Can you work these out from the model? Positions are in its coordinate system, mm. A direction names the side the tool comes from. Give positions to 0.01 mm unless a question says otherwise; leave off trailing zeros. Write each loop counter-clockwise with the first axis right and the second up, starting at its lowest first coordinate (ties: lowest second). Pieces come first, ordered by that corner, then holes. Notation, with made-up numbers: (32, 22.25) -> (44, 22.25) arc R15 ccw to (44, 35.25) -> close; hole circle Ø10 at (83.5, 72.5). An arc over 180 degrees is marked (long way). One line per item, written item: value.
from build123d import *

# Parameters (mm, degrees)
BOSS_EXTRUDE1_DEPTH     = 35
BOSS_EXTRUDE2_START     = 3
BOSS_EXTRUDE2_DEPTH     = 3
CUT_EXTRUDE1_DEPTH      = 54.037722425
CUT_EXTRUDE1_DEPTH_BACK = 54.037722425
CUT_EXTRUDE2_START      = -3
CUT_EXTRUDE2_DEPTH      = 6
CHAMFER1_SIZE           = 1


with BuildPart() as part:
    # Sketch1 → Boss-Extrude1 (new body)
    with BuildSketch(Plane(origin=(0, 0, 0), x_dir=(1, 0, 0), z_dir=(0, 1, 0))):
        with BuildLine():
            Line((7, 25.5), (7, 35.5))
            ThreePointArc((7, 35.5), (9.5, 38), (12, 35.5))
            Line((12, 35.5), (12, 10.5))
            ThreePointArc((12, 10.5), (11.827182716, 8.470776255), (11.313708499, 6.5))
            Line((11.313708499, 6.5), (8.013876853, -2.833333333))
            ThreePointArc((8.013876853, -2.833333333), (0, -8.5), (-8.013876853, -2.833333333))
            Line((-8.013876853, -2.833333333), (-11.313708499, 6.5))
            ThreePointArc((-11.313708499, 6.5), (-11.827182716, 8.470776255), (-12, 10.5))
            Line((-12, 10.5), (-12, 35.5))
            ThreePointArc((-12, 35.5), (-9.5, 38), (-7, 35.5))
            Line((-7, 35.5), (-7, 25.5))
            ThreePointArc((-7, 25.5), (0, 18.5), (7, 25.5))
        make_face()
        with BuildLine():
            Line((-6.599663291, 8.166666667), (-3.299831646, -1.166666667))
            ThreePointArc((-3.299831646, -1.166666667), (0, -3.5), (3.299831646, -1.166666667))
            Line((3.299831646, -1.166666667), (6.599663291, 8.166666667))
            ThreePointArc((6.599663291, 8.166666667), (0, 17.5), (-6.599663291, 8.166666667))
        make_face(mode=Mode.SUBTRACT)
    extrude(amount=BOSS_EXTRUDE1_DEPTH)

    # Sketch2 → Boss-Extrude2 (add)
    with BuildSketch(Plane.XZ.offset(BOSS_EXTRUDE2_START)):
        with BuildLine():
            Line((-12, -10.5), (-12, -35.5))
            ThreePointArc((-12, -35.5), (-9.5, -38), (-7, -35.5))
            Line((-7, -35.5), (-7, -25.5))
            ThreePointArc((-7, -25.5), (0, -18.5), (7, -25.5))
            Line((7, -25.5), (7, -35.5))
            ThreePointArc((7, -35.5), (9.5, -38), (12, -35.5))
            Line((12, -35.5), (12, -10.5))
            ThreePointArc((12, -10.5), (11.827182716, -8.470776255), (11.313708499, -6.5))
            Line((11.313708499, -6.5), (8.013876853, 2.833333333))
            ThreePointArc((8.013876853, 2.833333333), (0, 8.5), (-8.013876853, 2.833333333))
            Line((-8.013876853, 2.833333333), (-11.313708499, -6.5))
            ThreePointArc((-11.313708499, -6.5), (-11.827182716, -8.470776255), (-12, -10.5))
        make_face()
    extrude(amount=-BOSS_EXTRUDE2_DEPTH)

    # Sketch4 → Cut-Extrude1 (cut, two sides: drawn at the far end of the back side and taken through both)
    with BuildSketch(Plane(origin=(0, 0, 0), x_dir=(0, 0, -1), z_dir=(1, 0, 0)).offset(-CUT_EXTRUDE1_DEPTH_BACK)):
        with BuildLine():
            Line((21.5, 19), (31.5, 19))
            ThreePointArc((31.5, 19), (34.5, 16), (31.5, 13))
            Line((31.5, 13), (21.5, 13))
            ThreePointArc((21.5, 13), (18.5, 16), (21.5, 19))
        make_face()
    extrude(amount=CUT_EXTRUDE1_DEPTH + CUT_EXTRUDE1_DEPTH_BACK, mode=Mode.SUBTRACT)

    # Sketch5 → Cut-Extrude2 (cut)
    with BuildSketch(Plane(origin=(0, 16, 0), x_dir=(1, 0, 0), z_dir=(0, 1, 0)).offset(CUT_EXTRUDE2_START)):
        with BuildLine():
            Line((-11, 21.5), (-25, 21.5))
            Line((-25, 21.5), (-25, -28.5))
            Line((-25, -28.5), (25, -28.5))
            Line((25, -28.5), (25, 21.5))
            Line((25, 21.5), (11, 21.5))
            Line((11, 21.5), (11, 10.5))
            ThreePointArc((11, 10.5), (10.841584156, 8.639878234), (10.370899457, 6.833333333))
            Line((10.370899457, 6.833333333), (7.071067812, -2.5))
            ThreePointArc((7.071067812, -2.5), (0, -7.5), (-7.071067812, -2.5))
            Line((-7.071067812, -2.5), (-10.370899457, 6.833333333))
            ThreePointArc((-10.370899457, 6.833333333), (-10.841584156, 8.639878234), (-11, 10.5))
            Line((-11, 10.5), (-11, 21.5))
        make_face()
    extrude(amount=CUT_EXTRUDE2_DEPTH, mode=Mode.SUBTRACT)

    # Chamfer1
    chamfer1_edges = [part.edges().sort_by_distance(p)[0] for p in [
        (11, 19, -16),
        (10.841584156, 19, -8.639878234),
        (0, 19, 7.5),
        (-10.841584156, 19, -8.639878234),
        (-11, 13, -16),
        (-8.720983635, 13, -2.166666667),
        (8.720983635, 13, -2.166666667),
        (11, 13, -16),
        (-11, 19, -16),
        (-8.720983635, 19, -2.166666667),
        (0, 13, 7.5),
        (8.720983635, 19, -2.166666667),
        (10.841584156, 13, -8.639878234),
        (-10.841584156, 13, -8.639878234),
    ]]
    chamfer(chamfer1_edges, length=CHAMFER1_SIZE - 0.0001)  # a hair under: the kernel refuses the full size


solid = part.part
1) I need wall thicknesses on L1, parallel to Y at x = -8.5, z = -25; L2, parallel to X at y = 1, z = -25.5; L3, parallel to Y at x = -3.5, z = -8.5. Which ranges of each line are inside material? Lowest first, please.
Answer list:
L1: y = -3 to 13, 19 to 35
L2: x = -12 to -7, 7 to 12
L3: y = -3 to 0
2) If we section it at C-C (z = -33.5): Write out the boundary of the cut face in (x, y).
Answer list:
outline: (-12, -3) -> (-7, -3) -> (-7, 13.76) -> (-12, 13.76) -> close; (-12, 18.24) -> (-7, 18.24) -> (-7, 35) -> (-12, 35) -> close; (7, -3) -> (12, -3) -> (12, 13.76) -> (7, 13.76) -> close; (7, 18.24) -> (12, 18.24) -> (12, 35) -> (7, 35) -> close
3) Will these pins go through, and if not, where does the flat tip stop? pin 1 (4 mm diameter, centred on x = -5.5, y = 25, fed in from -Z); pin 2 (1.2 mm diameter, centred on y = 17, z = -13.5, fed in from -X); pin 3 (7 mm diameter, centred on x = 0, z = -7.5, fed in from +Y).
Answer list:
pin 1: stops at z = -37
pin 2: stops at x = -11
pin 3: stops at y = 0
4) If we section it at A-A (y = 4): Write out the boundary of the cut face in (x, z), and give its area (3 significant figures).
Answer list:
outline: (-12, -35.5) arc R2.5 ccw to (-7, -35.5) -> (-7, -25.5) arc R7 cw to (7, -25.5) -> (7, -35.5) arc R2.5 ccw to (12, -35.5) -> (12, -10.5) arc R12 ccw to (11.31, -6.5) -> (8.01, 2.83) arc R8.5 ccw to (-8.01, 2.83) -> (-11.31, -6.5) arc R12 ccw to (-12, -10.5) -> close; hole (-6.6, -8.17) arc R7 ccw (long way) to (6.6, -8.17) -> (3.3, 1.17) arc R3.5 ccw to (-3.3, 1.17) -> close
area: 531 mm^2
5) For faces 1 (the face through (-11.34, 13.49, -8.53)), 2 (the face through (10.846, 15.972, -8.666)), 3 (the face through (-7.2, 19, -26.4)), 4 (the face through (0.187, 17.255, -17.497)), which set-ups out of +Z, -Z, +X, -X, +Y, -Y let a thin tool reach every point of the face, with its end or its side?
Answer list:
face 1: +Z, -X
face 2: +Z, +X
face 3: +X, -X
face 4: +Y
6) We'd pull the mould along Z, two halves only. Please class faces 5 (the face through (7.2, 15.9, -18.5)), 6 (the face through (0.1, 16, 7.5)), 7 (the face through (-9.6, 15.7, -38)): released by +Z, released by -Z, zero draft, split by the parting line, or undercut.
Answer list:
face 5: undercut
face 6: released by +Z
face 7: released by -Z
7) If we section it at D-D (y = -1): Write out the boundary of the cut face in (x, z).
Answer list:
outline: (-12, -35.5) arc R2.5 ccw to (-7, -35.5) -> (-7, -25.5) arc R7 cw to (7, -25.5) -> (7, -35.5) arc R2.5 ccw to (12, -35.5) -> (12, -10.5) arc R12 ccw to (11.31, -6.5) -> (8.01, 2.83) arc R8.5 ccw to (-8.01, 2.83) -> (-11.31, -6.5) arc R12 ccw to (-12, -10.5) -> close
